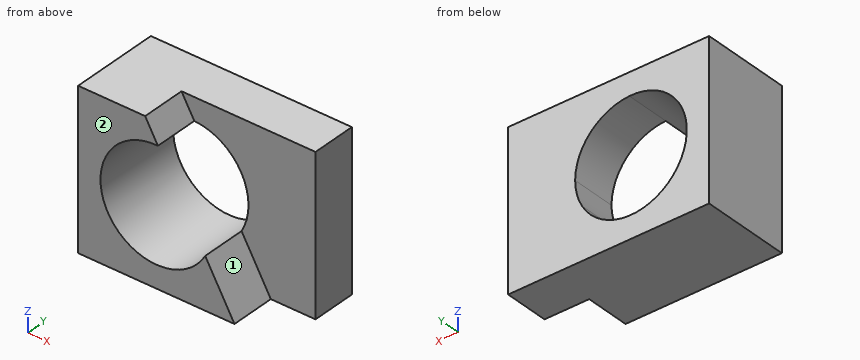
from build123d import *

# Parameters (mm, degrees)
F0_W     = 57.15
F0_H     = 44.45
F2_DEPTH = 25.4
F4_DEPTH = 12.7
F6_DEPTH = 25.4


with BuildPart() as f2:
    # F0 (on Front) → F2 (new body)
    with BuildSketch(Plane.XZ):
        with Locations((28.575, 22.225)):
            Rectangle(F0_W, F0_H)
    extrude(amount=F2_DEPTH)

    # F3 (on face) → F4 (cut)
    with BuildSketch(Plane.XZ.offset(25.4)):
        Polygon((19.05, 44.45), (44.45, 0), (57.15, 0), (57.15, 44.45), align=None)
    extrude(amount=-F4_DEPTH, mode=Mode.SUBTRACT)

    # F5 (on face) → F6 (cut)
    with BuildSketch(Plane.XZ.offset(25.4)):
        with BuildLine():
            ThreePointArc((36.128433, 14.562743), (37.599209, 18.269078), (38.1, 22.225))
            ThreePointArc((38.1, 22.225), (33.610865, 33.287446), (22.682337, 38.093411))
            Line((22.682337, 38.093411), (36.128433, 14.562743))
        make_face()
        with BuildLine():
            Line((36.128433, 14.562743), (22.682337, 38.093411))
            ThreePointArc((22.682337, 38.093411), (8.44164, 14.348794), (36.128433, 14.562743))
        make_face()
    extrude(amount=-F6_DEPTH, mode=Mode.SUBTRACT)


solid = f2.part
Part model, mm, in its own coordinate system. Face numbers are marked on the shaded views. A direction names the side the tool comes from. Coordinates: 2 decimals unless noted, no trailing zeros. Order: outer loops, then holes, each group sorted by start corner. A loop starts at its lowest first (then second) coordinate and runs counter-clockwise, first axis right, second up. Notation, with made-up numbers: M -10,47.5 L 0,47.5 A17 ccw 0,72.5 Z; hole C 80.5,51 d9. An arc over 180 degrees is marked long. One line per question, with ' | ' between items.
Q1. 3-axis set-ups, long thin cutter, end or side, ignore diameter. For the marked faces 1 and 2: which of +Z, -Z, +X, -X, +Y, -Y reach the whole face in a straight line?
A:
face 1: +Z, +X, -Y | face 2: +Z, -Z, +X, -X, -Y
Q2. Slice it at D-D (y = -23.25). Give the cut face in (x, z) (3 decimals).
A:
outline: M 0,0 L 44.45,0 L 36.128,14.563 A15.875 cw long 22.682,38.093 L 19.05,44.45 L 0,44.45 Z
Q3. Drill centre lines: line 1 (Y direction, x = 54, z = 31); line 2 (X direction, y = -9.5, z = 23.5); line 3 (X direction, y = -3.75, z = 24.5). Where is each one in solid material? Low to high.
A:
line 1: y = -12.7 to 0 | line 2: x = 0 to 6.4, 38.05 to 57.15 | line 3: x = 0 to 6.51, 37.94 to 57.15
Q4. Slice it at B-B (z = 35). Give the cut face in (x, y), and give its area (3 significant figures).
A:
outline: M 0,-25.4 L 12.8,-25.4 L 12.8,0 L 0,0 Z; M 31.65,-12.7 L 57.15,-12.7 L 57.15,0 L 31.65,0 Z | area: 649 mm^2
Q5. Slice it at A-A (y = -11). Give the cut face in (x, z) (3 decimals), and give its area (3 significant figures).
A:
outline: M 0,0 L 57.15,0 L 57.15,44.45 L 0,44.45 Z; hole M 36.128,14.563 A15.875 ccw 38.1,22.225 A15.875 ccw long Z | area: 1,750 mm^2
Q6. Pin check, flat tips, straight feed: P1, Ø1.5, axis at x = 6.5, z = 11.5, coming from the +Y side; P2, Ø2, axis at y = -16.5, z = 12.5, coming from the +X side; P3, Ø1.5, axis at x = 51, z = 37, coming from the -Y side. Stop position of each tip, or through.
A:
P1: stops at y = 0 | P2: stops at x = 37.88 | P3: stops at y = -12.7
Q7. Slice it at C-C (x = 8). Give the cut face in (y, z).
A:
outline: M -25.4,0 L 0,0 L 0,15.18 L -25.4,15.18 Z; M -25.4,29.27 L 0,29.27 L 0,44.45 L -25.4,44.45 Z
